```python
from build123d import *

# Parameters (mm, degrees)
F0_W          = 44.45
F0_H          = 44.45
F1_DEPTH      = 457.2
F5_DEPTH      = 25.4
F5_DEPTH_BACK = 24.638
F8_W          = 152.4
F8_H          = 152.4
F9_DEPTH      = 24.638
F9_DEPTH_BACK = 25.4


with BuildPart() as f1:
    # F0 (on Top) → F1 (new body)
    with BuildSketch(Plane.XY):
        with BuildLine():
            ThreePointArc((25.4, 22.225), (24.4700640303, 24.4700640303), (22.225, 25.4))
            Line((22.225, 25.4), (-22.225, 25.4))
            ThreePointArc((-22.225, 25.4), (-24.4700640303, 24.4700640303), (-25.4, 22.225))
            Line((-25.4, 22.225), (-25.4, -22.225))
            ThreePointArc((-25.4, -22.225), (-24.4700640303, -24.4700640303), (-22.225, -25.4))
            Line((-22.225, -25.4), (22.225, -25.4))
            ThreePointArc((22.225, -25.4), (24.4700640303, -24.4700640303), (25.4, -22.225))
            Line((25.4, -22.225), (25.4, 22.225))
        make_face()
        Rectangle(F0_W, F0_H, mode=Mode.SUBTRACT)
    extrude(amount=F1_DEPTH)

    # F4 (on face) → F5 (cut, two sides)
    with BuildSketch(Plane(origin=(161.6446101792, 161.6446101792, 228.6), x_dir=(0.8660254038, -0.2886751346, -0.4082482905), z_dir=(-0.5, -0.5, -0.7071067812))) as f5_sk:
        Polygon((-110.453744999, 187.8757004726), (-186.653744999, 264.0757004726), (-262.853744999, 340.2757004726), (-262.853744999, 187.8757004726), align=None)
        Polygon((-262.853744999, 340.2757004726), (-186.653744999, 264.0757004726), (-110.453744999, 187.8757004726), (-110.453744999, 340.2757004726), align=None)
    extrude(amount=-F5_DEPTH, mode=Mode.SUBTRACT)
    extrude(f5_sk.sketch, amount=F5_DEPTH_BACK, mode=Mode.SUBTRACT)

    # F8 (on face) → F9 (cut, two sides)
    with BuildSketch(Plane(origin=(0, 0, 0), x_dir=(0.9703149544, 0.0602782519, 0.2342123429), z_dir=(0.2418447626, -0.2418447626, -0.9396926208))) as f9_sk:
        Rectangle(F8_W, F8_H)
    extrude(amount=-F9_DEPTH, mode=Mode.SUBTRACT)
    extrude(f9_sk.sketch, amount=F9_DEPTH_BACK, mode=Mode.SUBTRACT)


solid = f1.part
```
Build history of the part. All positions in model axes, mm. A direction names the side the tool comes from. Coordinates: 2 decimals unless noted, no trailing zeros. Order: outer loops, then holes, each group sorted by start corner. A loop starts at its lowest first (then second) coordinate and runs counter-clockwise, first axis right, second up. Notation, with made-up numbers: (17, 16.25) -> (65, 16.25) arc R28 cw to (65, 38.25) -> close; hole circle Ø1 at (-29, 23). An arc over 180 degrees is marked (long way). Answer in a Markdown table with one row per item. Add a question column.
Q1. Which spindle directions (+Z, -Z, +X, -X, +Y, -Y) get a long thin tool onto all of the face, cutting with end or side? Do faces 4 (the face through (0, -22.225, 237)), 5 (the face through (0, -25.4, 239)). Say none if no direction does.
Q2. Band-saw the part on C-C, the plane z = 72. List the corners of the cut face in (x, y) (3 decimals), then the cut area to 3 significant figures.
Q3. Mould opens along X. For faces 1 (the face through (22.46, -7.64, 411.88)), 2 (the face through (0, 22.225, 216)), 3 (the face through (0, 25.4, 214)) say: +X half, -X half, draft (parallel to the pull), parting line (faces both ways), or undercut.
Q4. Band-saw the part on B-B, the plane y = -10.5. List the corners of the cut face in (x, z) (1 decimal).
Q5. Wall check: line 1 along Y through (x, z) = (15, 363.5) (3 decimals); line 2 along Y through (x, z) = (21.5, 36) (3 decimals). Give the ranges that are in metal, low to high. Write a range as [from, to].
Q6. Band-saw the part on A-A, the plane x = -11.5. List the corners of the cut face in (y, z) (3 decimals), then the cut area to 3 significant figures.
Q7. Band-saw the part on D-D, the plane z = 397. List the corners of the cut face in (x, y) (3 decimals).
Answers follow:
| question | item | result |
|---|---|---|
| 1 | face 4 | +Z, -Z |
| 1 | face 5 | +Z, -Z, +X, -X, -Y |
| 2 | outline | (-25.4, -22.225) arc R3.175 ccw to (-22.225, -25.4) -> (22.225, -25.4) arc R3.175 ccw to (25.4, -22.225) -> (25.4, 22.225) arc R3.175 ccw to (22.225, 25.4) -> (-22.225, 25.4) arc R3.175 ccw to (-25.4, 22.225) -> close; hole (-22.225, -22.225) -> (22.225, -22.225) -> (22.225, 22.225) -> (-22.225, 22.225) -> close |
| 2 | area | 596 mm^2 |
| 3 | face 1 | +X half |
| 3 | face 2 | undercut |
| 3 | face 3 | draft |
| 4 | outline | (-25.4, 22.4) -> (-22.2, 23.2) -> (-22.2, 445.5) -> (-25.4, 447.7) -> close; (22.2, 34.6) -> (25.4, 35.5) -> (25.4, 411.8) -> (22.2, 414.1) -> close |
| 5 | line 1 | [-25.4, -22.225], [22.225, 25.4] |
| 5 | line 2 | [22.225, 25.4] |
| 6 | outline | (-25.4, 29.797) -> (-22.225, 28.979) -> (-22.225, 446.204) -> (-25.4, 448.449) -> close; (22.225, 17.54) -> (25.4, 16.722) -> (25.4, 412.528) -> (22.225, 414.773) -> close |
| 6 | area | 2,590 mm^2 |
| 7 | outline | (-25.4, -22.225) arc R3.175 ccw to (-22.225, -25.4) -> (22.225, -25.4) arc R3.175 ccw to (25.4, -22.225) -> (25.4, 10.46) -> (22.225, 13.635) -> (22.225, -22.225) -> (-22.225, -22.225) -> (-22.225, 22.225) -> (13.635, 22.225) -> (10.46, 25.4) -> (-22.225, 25.4) arc R3.175 ccw to (-25.4, 22.225) -> close |
